```python
from build123d import *

# Parameters (mm, degrees)
SKETCH_2_R      = 1.5
EXTRUDE_1_DEPTH = 1.5
SKETCH_3_R      = 3.3
SKETCH_3_R_2    = 1.5
EXTRUDE_2_DEPTH = 1


with BuildPart() as part:
    # 草图2 → 凸台-拉伸1 (new body)
    with BuildSketch(Plane.XY):
        Polygon((-47.229146383, 20.256789608), (32.770853617, 20.256789608), (32.770853617, -19.743210392), (10.270853617, -19.743210392), (10.270853617, -56.743210392), (-24.729146383, -56.743210392), (-24.729146383, -19.743210392), (-47.229146383, -19.743210392), align=None)
        with Locations((-22.479146383, 15.506789608)):
            Circle(SKETCH_2_R, mode=Mode.SUBTRACT)
        with Locations(Location((8.020853617, 15.506789608, 0), (0, 0, 180))):
            Circle(SKETCH_2_R, mode=Mode.SUBTRACT)
        with Locations((8.020853617, -14.993210392)):
            Circle(SKETCH_2_R, mode=Mode.SUBTRACT)
        with Locations(Location((-22.479146383, -14.993210392, 0), (0, 0, 180))):
            Circle(SKETCH_2_R, mode=Mode.SUBTRACT)
        with Locations(Location((-21.979146383, -24.493210392, 0), (0, 0, 180))):
            Circle(SKETCH_2_R, mode=Mode.SUBTRACT)
        with Locations(Location((7.520853617, -24.493210392, 0), (0, 0, 180))):
            Circle(SKETCH_2_R, mode=Mode.SUBTRACT)
        with Locations(Location((-21.979146383, -53.993210392, 0), (0, 0, 180))):
            Circle(SKETCH_2_R, mode=Mode.SUBTRACT)
        with Locations(Location((7.520853617, -53.993210392, 0), (0, 0, 180))):
            Circle(SKETCH_2_R, mode=Mode.SUBTRACT)
        Polygon((-7.229146383, -7.743210392), (0.770853617, -7.743210392), (0.770853617, 8.256789608), (-15.229146383, 8.256789608), (-15.229146383, -7.743210392), align=None, mode=Mode.SUBTRACT)
    extrude(amount=EXTRUDE_1_DEPTH)

    # 草图3 → 凸台-拉伸2 (add)
    # profile 1 of 4: a face of its own
    with BuildSketch(Plane.XY.offset(1.5)):
        with Locations((-22.479146383, 15.506789608)):
            Circle(SKETCH_3_R)
        with Locations((-22.479146383, 15.506789608)):
            Circle(SKETCH_3_R_2, mode=Mode.SUBTRACT)
    # profile 2 of 4: a face of its own
    with BuildSketch(Plane.XY.offset(1.5)):
        with Locations((8.020853617, 15.506789608)):
            Circle(SKETCH_3_R)
        with Locations(Location((8.020853617, 15.506789608, 0), (0, 0, 180))):
            Circle(SKETCH_3_R_2, mode=Mode.SUBTRACT)
    # profile 3 of 4: a face of its own
    with BuildSketch(Plane.XY.offset(1.5)):
        with Locations((-22.479146383, -14.993210392)):
            Circle(SKETCH_3_R)
        with Locations(Location((-22.479146383, -14.993210392, 0), (0, 0, 180))):
            Circle(SKETCH_3_R_2, mode=Mode.SUBTRACT)
    # profile 4 of 4: a face of its own
    with BuildSketch(Plane.XY.offset(1.5)):
        with Locations((8.020853617, -14.993210392)):
            Circle(SKETCH_3_R)
        with Locations((8.020853617, -14.993210392)):
            Circle(SKETCH_3_R_2, mode=Mode.SUBTRACT)
    extrude(amount=EXTRUDE_2_DEPTH)


solid = part.part
```
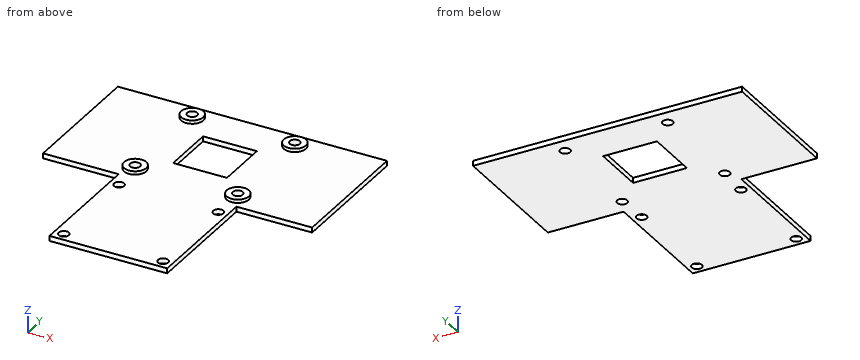
The model under review builds one solid part; all positions refer to its coordinate system, in mm. Coordinates: 2 decimals unless noted, no trailing zeros. Write each loop counter-clockwise with the first axis right and the second up, starting at its lowest first coordinate (ties: lowest second). Pieces come first, ordered by that corner, then holes.
1) We need section D-D on y = -43. State the section outline as (x, z) points, then the cut area to 3 significant figures.
2) We need section A-A on x = -2. State the section outline as (y, z) points, then the cut area to 3 significant figures.
3) We need section C-C on x = -22.5. State the section outline as (y, z) points.
4) To check wall thickness, follow probe 1 along X at (y, z) = (-16, 0.85); probe 2 along X at (y, z) = (-5.5, 0.35); probe 3 along X at (y, z) = (-23.5, 1.4). State the ranges of each line that lie inside material, in increasing order.
5) Clearance check with flat-ended pins moving along their axes: pin 1 Ø0.8 at (y, z) = (-43.5, 1) entering from +X; pin 2 Ø0.8 at (y, z) = (-46.5, 1) entering from -X. State where each tip first meets the part, or that it passes through.
6) We need section B-B on z = 0.4. Count the separate pieces of the cut face and the enclosed holes in it, then the cut area to 3 significant figures.
Answer list:
1. outline: (-24.73, 0) - (10.27, 0) - (10.27, 1.5) - (-24.73, 1.5) - close
1. area: 52.5 mm2
2. outline: (-56.74, 0) - (-7.74, 0) - (-7.74, 1.5) - (-56.74, 1.5) - close; (8.26, 0) - (20.26, 0) - (20.26, 1.5) - (8.26, 1.5) - close
2. area: 91.5 mm2
3. outline: (-56.74, 0) - (-55.4, 0) - (-55.4, 1.5) - (-56.74, 1.5) - close; (-52.59, 0) - (-25.9, 0) - (-25.9, 1.5) - (-52.59, 1.5) - close; (-23.09, 0) - (-16.49, 0) - (-16.49, 2.5) - (-18.29, 2.5) - (-18.29, 1.5) - (-23.09, 1.5) - close; (-13.49, 0) - (14.01, 0) - (14.01, 2.5) - (12.21, 2.5) - (12.21, 1.5) - (-11.69, 1.5) - (-11.69, 2.5) - (-13.49, 2.5) - close; (17.01, 0) - (20.26, 0) - (20.26, 1.5) - (18.81, 1.5) - (18.81, 2.5) - (17.01, 2.5) - close
4. probe 1: x = -47.23 to -23.59, -21.37 to 6.91, 9.13 to 32.77
4. probe 2: x = -47.23 to -15.23, 0.77 to 32.77
4. probe 3: x = -24.73 to -23.1, -20.86 to 6.4, 8.64 to 10.27
5. pin 1: stops at x = 10.27
5. pin 2: stops at x = -24.73
6. separate pieces: 1
6. enclosed holes: 9
6. area: 4,180 mm2
